from build123d import *

# Parameters (mm, degrees)
SKETCH1_R           = 4.445
BOSS_EXTRUDE1_DEPTH = 5.08
SKETCH2_R           = 3.81
BOSS_EXTRUDE2_DEPTH = 0.635
BOSS_EXTRUDE2_TAPER = 15
CUT_EXTRUDE1_START  = -1.27
SKETCH3_R           = 4.445
SKETCH3_R_2         = 4.1275
CUT_EXTRUDE1_DEPTH  = 1.27
CHAMFER1_SIZE       = 0.381
CUT_EXTRUDE2_DEPTH  = 9.495721049


with BuildPart() as part:
    # Sketch1 → Boss-Extrude1 (new body)
    with BuildSketch(Plane.XY):
        Circle(SKETCH1_R)
    extrude(amount=BOSS_EXTRUDE1_DEPTH)

    # Sketch2 → Boss-Extrude2 (add)
    with BuildSketch(Plane(origin=(0, 0, 0), x_dir=(-1, 0, 0), z_dir=(0, 0, -1))):
        Circle(SKETCH2_R)
    extrude(amount=BOSS_EXTRUDE2_DEPTH, taper=BOSS_EXTRUDE2_TAPER)

    # Sketch3 → Cut-Extrude1 (cut)
    with BuildSketch(Plane.XY.offset(5.08).offset(CUT_EXTRUDE1_START)):
        Circle(SKETCH3_R)
        Circle(SKETCH3_R_2, mode=Mode.SUBTRACT)
    extrude(amount=CUT_EXTRUDE1_DEPTH, mode=Mode.SUBTRACT)

    # Chamfer1
    chamfer1_edges = [part.edges().sort_by_distance(p)[0] for p in [
        (-4.1275, 0, 5.08),
    ]]
    chamfer(chamfer1_edges, length=CHAMFER1_SIZE)

    # Sketch5 → Cut-Extrude2 (cut, through all)
    with BuildSketch(Plane.XY.offset(5.08)):
        Polygon((-1.374815329, 2.38125), (-2.749630657, 0), (-1.374815329, -2.38125), (1.374815329, -2.38125), (2.749630657, 0), (1.374815329, 2.38125), align=None)
    extrude(amount=-CUT_EXTRUDE2_DEPTH, mode=Mode.SUBTRACT)


solid = part.part
Input: part model. Units: mm. Frame: model coordinates. A direction names the side the tool comes from. Give positions to 0.01 mm unless a question says otherwise; leave off trailing zeros. Write each loop counter-clockwise with the first axis right and the second up, starting at its lowest first coordinate (ties: lowest second). Pieces come first, ordered by that corner, then holes. Notation, with made-up numbers: (25, 59.5) -> (73, 59.5) arc R31 ccw to (73, 91.5) -> close; hole circle Ø7 at (73, 25.5). An arc over 180 degrees is marked (long way). Use one line per item in the form item = value. Start each with the question number.
1) Pin query (flat end, axial travel): pin 1 (1 mm diameter, centred on y = 3.5, z = 2, fed in from -X); pin 2 (2 mm diameter, centred on x = 2, z = 0.5, fed in from -Y). Return the tip coordinate at first contact, or that it passes through.
2) Section query C-C on z = 1.7. Return the cut outline in (x, y) (3 decimals).
3) Section query B-B on z = 4.45. Return the cut outline in (x, y) (1 decimal), then the cut area to 3 significant figures.
4) Draft query along X for faces 4 (the cylindrical face through (-0.96, -4.34, 1.88)), 5 (the flat face through (2.5, 0.9, -0.635)), 6 (the flat face through (0, 2.381, 2)). Return one class per face: pulls with the +X half, pulls with the -X half, needs draft (parallel to the pull), parting line crosses it, or undercut.
5) Ray query, probe 1 along Y at (x, z) = (-2.25, 3.6); probe 2 along Y at (x, z) = (-2.5, 2.7); probe 3 along X at (y, z) = (2.25, 0.7). Return the intervals inside material, ascending. Write a range as from..to.
6) Set-up query: faces 1 (the flat face through (4, 1, 0)), 2 (the flat face through (-2.072, -1.174, 2.263)), 3 (the cylindrical face through (3.937, 1.24, 4.248)). Return all of +Z, -Z, +X, -X, +Y, -Y with unobstructed straight access to the full face (end or side cutting, diameter ignored); none if empty.
Outcome:
q1.pin_1 = -3.28
q1.pin_2 = -4.33
q2.outline = circle Ø8.89 at (0, 0); hole (-2.75, 0) -> (-1.375, -2.381) -> (1.375, -2.381) -> (2.75, 0) -> (1.375, 2.381) -> (-1.375, 2.381) -> close
q3.outline = circle Ø8.3 at (0, 0); hole (-2.7, 0) -> (-1.4, -2.4) -> (1.4, -2.4) -> (2.7, 0) -> (1.4, 2.4) -> (-1.4, 2.4) -> close
q3.area = 33.9 mm^2
q4.face_4 = parting line crosses it
q4.face_5 = needs draft
q4.face_6 = undercut
q5.probe_1 = -3.83..-0.87, 0.87..3.83
q5.probe_2 = -3.68..-0.43, 0.43..3.68
q5.probe_3 = -3.83..-1.45, 1.45..3.83
q6.face_1 = -Z
q6.face_2 = +Z, -Z
q6.face_3 = +Z
